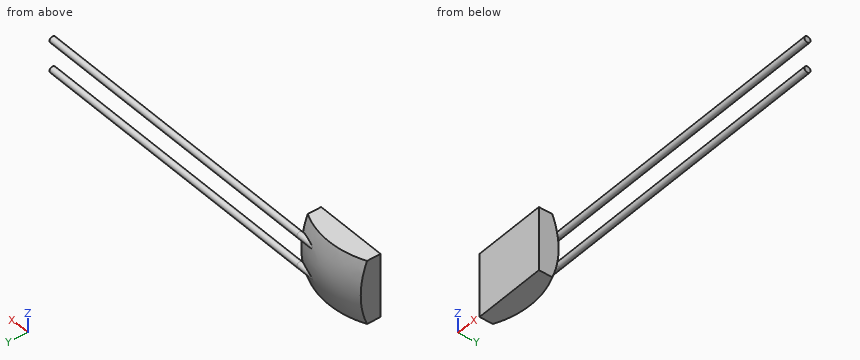
from build123d import *

# Parameters (mm, degrees)
SKETCH_3_OUTSIDE_W   = 6.506
SKETCH_3_OUTSIDE_H   = 6.506
SKETCH_3_OUTSIDE_W_2 = 2.4
SKETCH_3_OUTSIDE_H_2 = 2.1
CUT_EXTRUDE_1_DEPTH  = 1.9
SKETCH_4_R           = 0.1
EXTRUDE_2_DEPTH      = 10
EXTRUDE_2_DEPTH_BACK = 1


with BuildPart() as part:
    # Эскиз2 → Повернуть1 (revolve)
    with BuildSketch(Plane.XY):
        with BuildLine():
            Line((0, 0), (1.75, 0))
            Line((1.75, 0), (1.75, 0.336698586))
            ThreePointArc((1.75, 0.336698586), (0.919212772, 0.755704445), (0, 0.9))
            Line((0, 0.9), (0, 0))
        make_face()
    revolve(axis=Axis((0, 0, 0), (0, 1, 0)))

    # Эскиз3 outside → Вырез-Вытянуть1 (cut, through all)
    with BuildSketch(Plane.XZ):
        Rectangle(SKETCH_3_OUTSIDE_W, SKETCH_3_OUTSIDE_H)
        Rectangle(SKETCH_3_OUTSIDE_W_2, SKETCH_3_OUTSIDE_H_2, mode=Mode.SUBTRACT)
    extrude(amount=-CUT_EXTRUDE_1_DEPTH, mode=Mode.SUBTRACT)

    # Эскиз4 → Бобышка-Вытянуть2 (add, two sides)
    with BuildSketch(Plane(origin=(1.2, 0, 0), x_dir=(0, 0, -1), z_dir=(1, 0, 0))) as extrude_2_sk:
        with Locations((-0.5, 0.7)):
            Circle(SKETCH_4_R)
        with Locations((0.5, 0.7)):
            Circle(SKETCH_4_R)
    extrude(amount=EXTRUDE_2_DEPTH)
    extrude(extrude_2_sk.sketch, amount=-EXTRUDE_2_DEPTH_BACK)


solid = part.part
Check sheet for the modelled part. Datum: model origin and axes. Units: mm. Round coordinates to 2 decimals unless told otherwise and drop trailing zeros. Loops run counter-clockwise (first coordinate to the right, second up) from the corner with the lowest first, then second, coordinate; pieces in that order, holes last.
1. Scan lines: probe 1 along Z at (x, y) = (8.25, 0.7); probe 2 along Y at (x, z) = (6, 0.5); probe 3 along X at (y, z) = (0.1, -0.8). Record each from-to range of solid material in increasing order.
2. Sectioned sample at C-C on z = -0.75. Record the boundary of the cut face in (x, y).
3. Sectioned sample at A-A on x = 8.25. Record the boundary of the cut face in (y, z), and give its area (3 significant figures).
4. Sectioned sample at B-B on y = 0.15. Record the boundary of the cut face in (x, z).
Recorded:
1. probe 1: z = -0.6 to -0.4, 0.4 to 0.6
1. probe 2: y = 0.6 to 0.8
1. probe 3: x = -1.2 to 1.2
2. outline: (-1.2, 0) - (1.2, 0) - (1.2, 0.55) arc R2.9 ccw to (-1.2, 0.55) - close
3. outline: circle Ø0.2 at (0.7, -0.5); circle Ø0.2 at (0.7, 0.5)
3. area: 0.0628 mm2
4. outline: (-1.2, -1.05) - (1.2, -1.05) - (1.2, 1.05) - (-1.2, 1.05) - close
